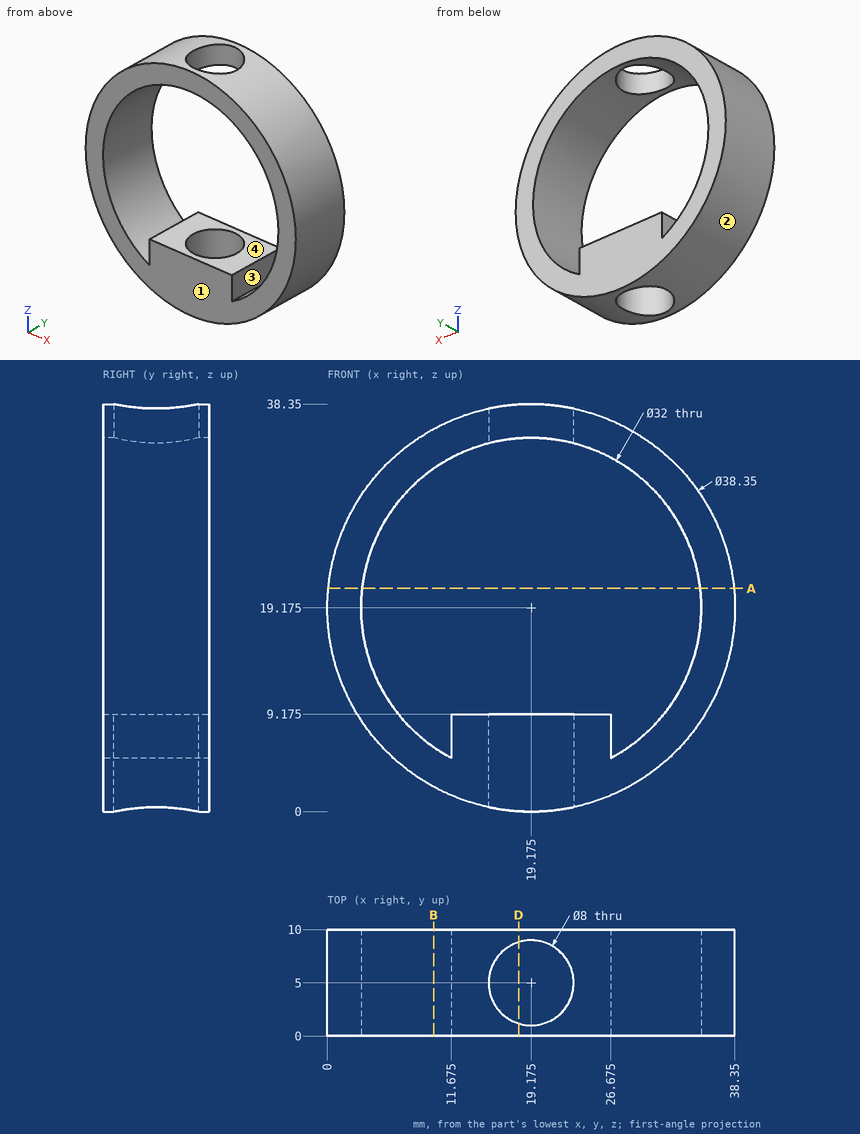
For this review, use the dimensioned drawing (mm, ordinates from the lowest corner) and the shaded views. Give positions to 0.01 mm unless a question says otherwise; leave off trailing zeros. Order: outer loops, then holes, each group sorted by start corner. A loop starts at its lowest first (then second) coordinate and runs counter-clockwise, first axis right, second up. Notation, with made-up numbers: M 2.25,-33 L 15.25,-33 A16 ccw 15.25,-13 Z; hole C 0.5,-26 d1. An arc over 180 degrees is marked long. Use one line per item in the form item = value. Start each with the question number.
Item 1: The part is to be moulded in two halves that separate along Z. For the marked faces 1, 2, 3 and 4, say which applies: pulls with the +Z half, pulls with the -Z half, needs draft (parallel to the pull), parting line crosses it, or undercut.
Item 2: To check wall thickness, follow line 1 along Z through (x, y) = (25, 6.5) (3 decimals); line 2 along Z through (x, y) = (9, 8.25); line 3 along X through (y, z) = (6, 35.5). State the ranges of each line that lie inside material, in increasing order. Write a range as from..to.
Item 3: Insertion check: pin 1 Ø1.2 at (y, z) = (5.5, 7) entering from +X; pin 2 Ø6 at (x, y) = (26, 5) entering from +Z; pin 3 Ø2 at (y, z) = (4.5, 7) entering from -X. Each pin has a flat end and moves straight along its axis. Give the tip position at first contact, or say it passes through.
Item 4: We need section A-A on z = 21. Give the boundary of the cut face in (x, y), plus the area to 3 significant figures.
Item 5: We need section B-B on x = 10. Give the boundary of the cut face in (y, z).
Item 6: We need section D-D on x = 18. Give the boundary of the cut face in (y, z) (3 decimals).
Completed:
q1.face_1 = needs draft
q1.face_2 = parting line crosses it
q1.face_3 = undercut
q1.face_4 = undercut
q2.line_1 = 0.906..9.175, 34.077..37.444
q2.line_2 = 2.92..6.83, 31.52..35.43
q2.line_3 = 9.12..15.3, 23.05..29.23
q3.pin_1 = 34.46
q3.pin_2 = 37.94
q3.pin_3 = 3.59
q4.outline = M 0.09,0 L 3.28,0 L 3.28,10 L 0.09,10 Z; M 35.07,0 L 38.26,0 L 38.26,10 L 35.07,10 Z
q4.area = 63.8 mm²
q5.outline = M 0,2.34 L 10,2.34 L 10,6.07 L 0,6.07 Z; M 0,32.28 L 10,32.28 L 10,36.01 L 0,36.01 Z
q6.outline = M 0,0.036 L 1.176,0.036 L 1.176,9.175 L 0,9.175 Z; M 0,35.132 L 1.176,35.132 L 1.176,38.314 L 0,38.314 Z; M 8.824,0.036 L 10,0.036 L 10,9.175 L 8.824,9.175 Z; M 8.824,35.132 L 10,35.132 L 10,38.314 L 8.824,38.314 Z
